Geometry check sheet. Reference: the model listing, model coordinates, mm. Coordinates: 2 decimals unless noted, no trailing zeros. Write each loop counter-clockwise with the first axis right and the second up, starting at its lowest first coordinate (ties: lowest second). Pieces come first, ordered by that corner, then holes. Notation, with made-up numbers: (28, 84) -> (51, 84) arc R6 cw to (51, 88) -> close; hole circle Ø7 at (63, 34). An arc over 180 degrees is marked (long way). Answer in a Markdown table with one row per item. Add a question column.
1. Cross-section at C-C on y = 27. Record the cut outline in (x, z).
2. Cross-section at A-A on z = 0. Record the cut outline in (x, y), and give its area (3 significant figures).
3. Depth check by flat-ended pin: P1, Ø12, axis at y = -2.5, z = 154.5, coming from the +X side; P2, Ø2, axis at x = 103, y = 45, coming from the -Z side; P3, Ø6, axis at x = -7, y = 35, coming from the -Z side. Enter the tip coordinate at first touch or a pass-through.
4. Scan lines: L1, parallel to Z at x = 0, y = -55; L2, parallel to X at y = -29, z = 46.5; L3, parallel to Z at x = 98, y = 61.5. Record each from-to range of solid material in increasing order. Write a range as from..to.
5. Cross-section at B-B on x = 0. Record the cut outline in (y, z).
```python
from build123d import *

# Parameters (mm, degrees)
F0_R          = 254
F0_R_2        = 203.2
F2_DEPTH      = 76.2
F2_DEPTH_BACK = 76.2
F3_R          = 19.05


# Not quite as in the source:
# - the program builds the solid bodies; features that only make, move or delete a surface that nothing else refers to are left out


with BuildPart() as f2:
    # F0 (on Front) → F2 (new body, two sides)
    with BuildSketch(Plane.XZ) as f2_sk:
        Circle(F0_R)
        Circle(F0_R_2, mode=Mode.SUBTRACT)
    extrude(amount=F2_DEPTH)
    extrude(f2_sk.sketch, amount=-F2_DEPTH_BACK)

    # F3
    f3_edges = [f2.edges().sort_by_distance(p)[0] for p in [
        (-254, 76.2, 0),
        (-254, -76.2, 0),
    ]]
    fillet(f3_edges, radius=F3_R)


solid = f2.part
```
Results found:
| question | item | result |
|---|---|---|
| 1 | outline | circle Ø508 at (0, 0); hole circle Ø406.4 at (0, 0) |
| 2 | outline | (-254, -57.15) arc R19.05 ccw to (-234.95, -76.2) -> (-203.2, -76.2) -> (-203.2, 76.2) -> (-234.95, 76.2) arc R19.05 ccw to (-254, 57.15) -> close; (203.2, -76.2) -> (234.95, -76.2) arc R19.05 ccw to (254, -57.15) -> (254, 57.15) arc R19.05 ccw to (234.95, 76.2) -> (203.2, 76.2) -> close |
| 2 | area | 15,200 mm^2 |
| 3 | P1 | stops at x = 206.07 |
| 3 | P2 | stops at z = -232.62 |
| 3 | P3 | stops at z = -253.97 |
| 4 | L1 | z = -254..-203.2, 203.2..254 |
| 4 | L2 | x = -249.71..-197.81, 197.81..249.71 |
| 4 | L3 | z = -233.79..-178.01, 178.01..233.79 |
| 5 | outline | (-76.2, -234.95) arc R19.05 ccw to (-57.15, -254) -> (57.15, -254) arc R19.05 ccw to (76.2, -234.95) -> (76.2, -203.2) -> (-76.2, -203.2) -> close; (-76.2, 203.2) -> (76.2, 203.2) -> (76.2, 234.95) arc R19.05 ccw to (57.15, 254) -> (-57.15, 254) arc R19.05 ccw to (-76.2, 234.95) -> close |
